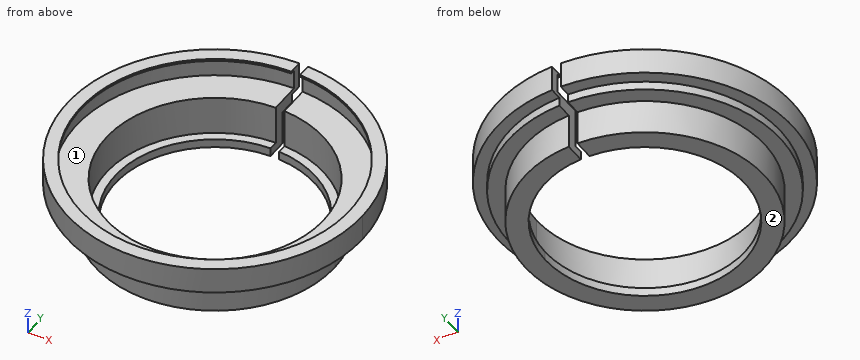
Autodesk Inventor part; units mm, degrees
ref_plane "YZ Plane" through (0, 0, 0) normal (1, 0, 0) x (0, 1, 0)
ref_plane "XZ Plane" through (0, 0, 0) normal (0, 1, 0) x (-1, 0, 0)
ref_plane "XY Plane" through (0, 0, 0) normal (0, 0, 1) x (1, 0, 0)
sketch "Sketch1" plane through (0, 0, 0) normal (0, 0, 1) x (1, 0, 0)
  circle A0 centre (0, 0) radius 13.8
  circle A1 centre (0, 0) radius 11.5
  circle A2 centre (0, 0) radius 15.6
  circle A3 centre (0, 0) radius 12.5
  dimension "d0" = 27.6
  dimension "d1" = 23
  dimension "d2" = 31.2
  dimension "d3" = 25
extrude "Extrusion1" add sketch "Sketch1" along normal blind 1 contours A3
extrude "Extrusion2" add sketch "Sketch1" along normal blind 4 contours A0
sketch "Sketch2" plane through (0, 0, 4) normal (0, 0, 1) x (1, 0, 0)
  circle A0 centre (0, 0) radius 15.6
  circle A1 centre (0, 0) radius 12.5
extrude "Extrusion3" add sketch "Sketch2" along normal blind 1
sketch "Sketch4" plane through (0, 0, 5) normal (0, 0, 1) x (1, 0, 0)
  circle A0 centre (0, 0) radius 16
  circle A1 centre (0, 0) radius 17
  circle A2 centre (0, 0) radius 12.5
  dimension "d14" = 32
  dimension "d15" = 34
extrude "Extrusion5" add sketch "Sketch4" along normal blind 0.5 contours A0
extrude "Extrusion6" add sketch "Sketch4" along normal blind 3 contours A1
sketch "Sketch5" plane through (0, 0, 8) normal (0, 0, 1) x (1, 0, 0)
  circle A0 centre (0, 0) radius 16
  circle A1 centre (0, 0) radius 15.5
  dimension "d20" = 31
extrude "Extrusion7" add sketch "Sketch5" against normal blind 0.25
sketch "Sketch8" plane through (0, 0, 8) normal (0, 0, 1) x (1, 0, 0)
  line L0 (0.5, 10) -> (-0.5, 10)
  line L1 (-0.5, 10) -> (-0.5, 20)
  line L2 (-0.5, 20) -> (0.5, 20)
  line L3 (0.5, 20) -> (0.5, 10)
  circle A0 centre (0, 0) radius 15
  line L4 (0.5, 10) -> (-0.5, 20) construction
  line L5 (-0.5, 10) -> (0.5, 20) construction
  point P0 (0, 15)
  dimension "d30" = 1
  dimension "d31" = 10
extrude "Extrusion10" cut sketch "Sketch8" against normal blind 10 contours L0 L1 A0 L3 | A0 L1 L2 L3 picked at (-0.0556, 11.6664)
properties part number "32to25mmFilterAdapter"
The model under review builds one solid part; all positions refer to its coordinate system, in mm. Face numbers are marked on the shaded views. Round coordinates to 2 decimals unless told otherwise and drop trailing zeros. Loops run counter-clockwise (first coordinate to the right, second up) from the corner with the lowest first, then second, coordinate; pieces in that order, holes last. Notation, with made-up numbers: (-22, 73) -> (23, 73) arc R19 ccw to (23, 108) -> close; hole circle Ø3 at (50.5, 76). An arc over 180 degrees is marked (long way). Answer as a JSON object with one key per item and string values. Group by question number.
1) We need section C-C on x = -10.5. Write out the cut boundary in (y, z), then the cut area to 3 significant figures.
2) We need section D-D on y = -14.5. Write out the cut boundary in (x, z).
3) We need section B-B on y = -1.5. Write out the cut boundary in (x, z).
4) For line 1 (X direction, y = 0, z = 0.25); line 2 (Y direction, x = 0, z = 7.3); line 3 (Y direction, x = 7.5, z = 6), list the stretches that pass through material, from the lowest coordinate up. Write a range as [from, to].
5) Mouldability with a two-part tool opening along Y and no side actions: class the marked faces 1 and 2 as released by +Y, released by -Y, zero draft, split by the parting line, or undercut.
6) We need section A-A on x = 0. Write out the cut boundary in (y, z), then the cut area to 3 significant figures.
7) For pin 1 Ø4 at (y, z) = (-10.5, 5.5) entering from +X; pin 2 Ø4 at (x, y) = (10.5, 12.5) entering from -Z; pin 3 Ø9.5 at (x, y) = (7.5, 6.5) entering from +Z; pin 4 Ø5 at (x, y) = (8.5, -10.5) entering from -Z, all flat-tipped, find the tip position at first contact; note any pin that passes through.
Result set:
{
 "1": {"outline": "(-13.37, 5) -> (-11.54, 5) -> (-11.54, 4) -> (-8.95, 4) -> (-8.95, 0) -> (-4.69, 0) -> (-4.69, 1) -> (-6.78, 1) -> (-6.78, 5.5) -> (-12.07, 5.5) -> (-12.07, 7.75) -> (-11.4, 7.75) -> (-11.4, 8) -> (-13.37, 8) -> close; (4.69, 0) -> (8.95, 0) -> (8.95, 4) -> (11.54, 4) -> (11.54, 5) -> (13.37, 5) -> (13.37, 8) -> (11.4, 8) -> (11.4, 7.75) -> (12.07, 7.75) -> (12.07, 5.5) -> (6.78, 5.5) -> (6.78, 1) -> (4.69, 1) -> close", "area": "44.5 mm²"},
 "2": {"outline": "(-8.87, 5) -> (-5.75, 5) -> (-5.75, 4) -> (5.75, 4) -> (5.75, 5) -> (8.87, 5) -> (8.87, 8) -> (5.48, 8) -> (5.48, 7.75) -> (6.76, 7.75) -> (6.76, 5.5) -> (-6.76, 5.5) -> (-6.76, 7.75) -> (-5.48, 7.75) -> (-5.48, 8) -> (-8.87, 8) -> close"},
 "3": {"outline": "(-16.93, 5) -> (-15.53, 5) -> (-15.53, 4) -> (-13.72, 4) -> (-13.72, 0) -> (-11.4, 0) -> (-11.4, 1) -> (-12.41, 1) -> (-12.41, 5.5) -> (-15.93, 5.5) -> (-15.93, 7.75) -> (-15.43, 7.75) -> (-15.43, 8) -> (-16.93, 8) -> close; (11.4, 0) -> (13.72, 0) -> (13.72, 4) -> (15.53, 4) -> (15.53, 5) -> (16.93, 5) -> (16.93, 8) -> (15.43, 8) -> (15.43, 7.75) -> (15.93, 7.75) -> (15.93, 5.5) -> (12.41, 5.5) -> (12.41, 1) -> (11.4, 1) -> close"},
 "4": {"line 1": "[-13.8, -11.5], [11.5, 13.8]", "line 2": "[-17, -16]", "line 3": "[-15.26, -14.13], [14.13, 15.26]"},
 "5": {"face 1": "undercut", "face 2": "zero draft"},
 "6": {"outline": "(-17, 5) -> (-15.6, 5) -> (-15.6, 4) -> (-13.8, 4) -> (-13.8, 0) -> (-11.5, 0) -> (-11.5, 1) -> (-12.5, 1) -> (-12.5, 5.5) -> (-16, 5.5) -> (-16, 7.75) -> (-15.5, 7.75) -> (-15.5, 8) -> (-17, 8) -> close", "area": "14.2 mm²"},
 "7": {"pin 1": "x = 14.72", "pin 2": "z = 4", "pin 3": "z = 5.5", "pin 4": "z = 0"}
}
